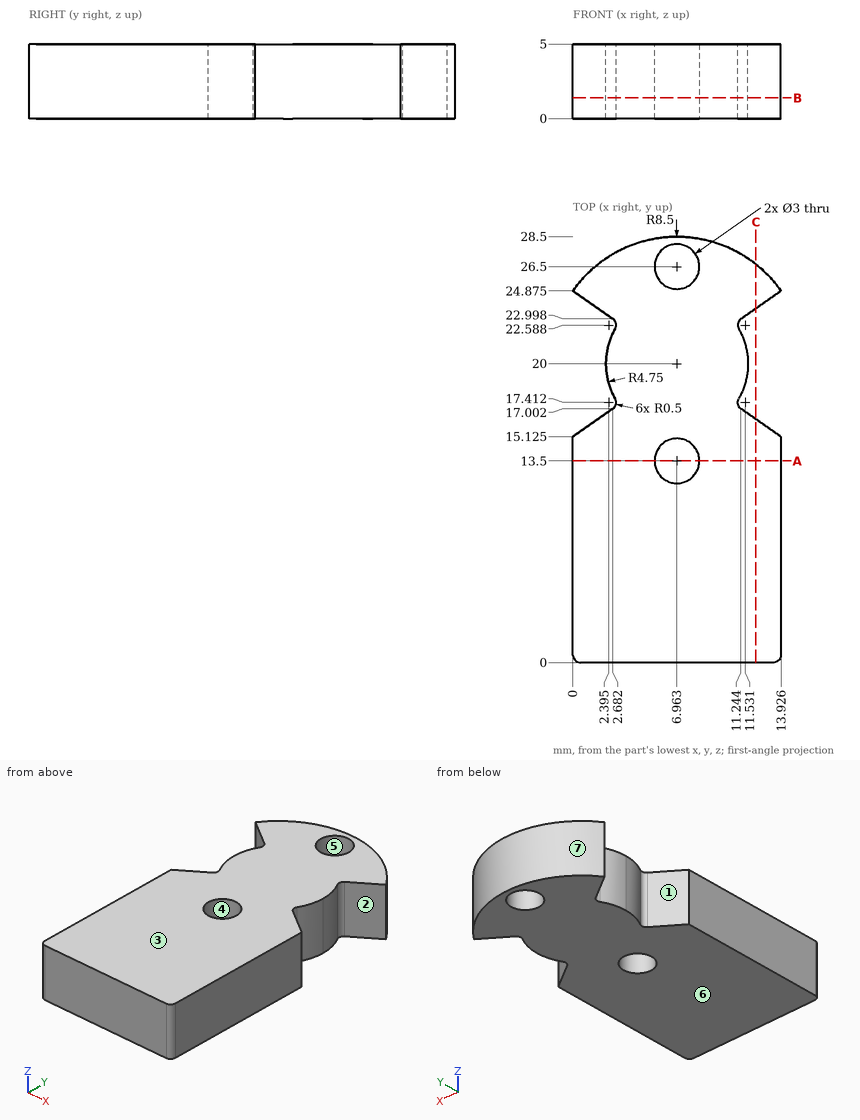
Study the drawing (mm; zero at the part's minimum x, y, z) and answer. A direction names the side the tool comes from. Give positions to 0.01 mm unless a question says otherwise; leave off trailing zeros. Loops run counter-clockwise (first coordinate to the right, second up) from the corner with the lowest first, then second, coordinate; pieces in that order, holes last. Notation, with made-up numbers: (-20, 51.5) -> (-14, 51.5) arc R30 cw to (-14, 79.5) -> close; hole circle Ø6 at (29, 30.5). An arc over 180 degrees is marked (long way). Use a Markdown table: item, result. Add a question column.
1) The part is cut by section C-C, the plane x = 12.25. Determine the outline of the cut face in (y, z) (1 decimal).
2) The part is cut by section B-B, the plane z = 1.4. Count the separate pieces of the cut face and the enclosed holes in it.
3) Which of the six approach directions +Z, -Z, +X, -X, +Y, -Y give full straight-line access (tool end or side, diameter ignored) to the marked faces 1, 2 and 3?
4) For a pull along X with two mould halves and no side action, classify the marked faces 4, 5, 6 and 7 as +X half, -X half, draft (parallel to the pull), parting line (faces both ways), or undercut.
5) Consider line 1 along Y through (x, z) = (5.75, 4.3) (1 decimal); line 2 along Y through (x, z) = (6.5, 3.15); line 3 along X through (y, z) = (20, 2.6). Determine where each line is inside the solid, lowest interval first.
6) The part is cut by section A-A, the plane y = 13.5. Determine the outline of the cut face in (x, z) (1 decimal).
7) This flat-tipped pin is pushed along its axis until it touches: P1, Ø1.8, axis at x = 6.96, y = 13.5, coming from the +Z side. Where does it stop, or does it pass through?
Reported:
| question | item | result |
|---|---|---|
| 1 | outline | (0, 0) -> (16.3, 0) -> (16.3, 5) -> (0, 5) -> close; (23.7, 0) -> (26.7, 0) -> (26.7, 5) -> (23.7, 5) -> close |
| 2 | separate pieces | 1 |
| 2 | enclosed holes | 2 |
| 3 | face 1 | +Z, -Z, -X |
| 3 | face 2 | +Z, -Z, +X |
| 3 | face 3 | +Z, +X, -X, +Y, -Y |
| 4 | face 4 | undercut |
| 4 | face 5 | undercut |
| 4 | face 6 | draft |
| 4 | face 7 | parting line |
| 5 | line 1 | y = 0 to 12.6, 14.4 to 25.6, 27.4 to 28.4 |
| 5 | line 2 | y = 0 to 12.07, 14.93 to 25.07, 27.93 to 28.49 |
| 5 | line 3 | x = 2.21 to 11.71 |
| 6 | outline | (0, 0) -> (5.5, 0) -> (5.5, 5) -> (0, 5) -> close; (8.5, 0) -> (13.9, 0) -> (13.9, 5) -> (8.5, 5) -> close |
| 7 | P1 | passes through |
